Input: dimensioned drawing with shaded views. Units: mm. Origin: part minimum x, y, z. A direction names the side the tool comes from. Round coordinates to 2 decimals unless told otherwise and drop trailing zeros. Order: outer loops, then holes, each group sorted by start corner. A loop starts at its lowest first (then second) coordinate and runs counter-clockwise, first axis right, second up. Notation, with made-up numbers: M -37,73 L 10,73 A15 cw 10,91 Z; hole C 85.5,21.25 d4. An arc over 180 degrees is marked long. Answer as CSV lines item,"result". Start each with the question number.
Item 1: Line query: line 1 (Z direction, x = 113, y = 8.75); line 2 (X direction, y = 7.25, z = 78); line 3 (Y direction, x = 22, z = 23.5). Output: solid intervals per line, ascending. Write a range as [from, to].
Item 2: Set-up query: the marked faces 1 and 2. Return all of +Z, -Z, +X, -X, +Y, -Y with unobstructed straight access to the full face (end or side cutting, diameter ignored); none if empty.
Item 3: Section query D-D on z = 21.5. Return the cut outline in (x, y).
Item 4: Section query C-C on x = 7. Return the cut outline in (y, z).
Item 5: First-contact query: P1, Ø1, axis at x = 7.5, z = 77, coming from the +Y side; P2, Ø3, axis at x = 7, z = 7, coming from the -Y side. Flat tips, straight axial feed; report the tip coordinate or a pass-through.
Item 6: Section query B-B on z = 7. Return the cut outline in (x, y).
Item 7: Section query A-A on y = 5.75. Return the cut outline in (x, z), plus the area to 3 significant figures.
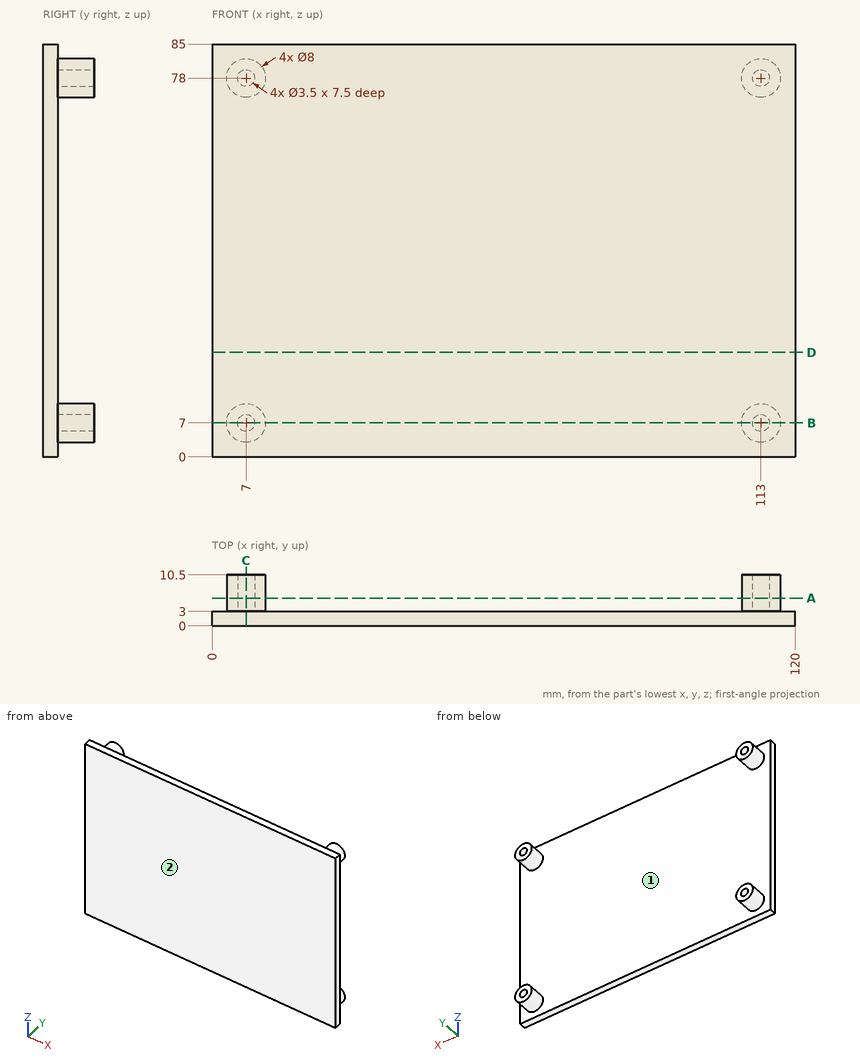
Results:
1,line 1,"[3, 5.25], [8.75, 11], [74, 76.25], [79.75, 82]"
1,line 2,"[3, 5.25], [8.75, 11], [109, 111.25], [114.75, 117]"
1,line 3,"[0, 3]"
2,face 1,"+Y"
2,face 2,"+Z, -Z, +X, -X, -Y"
3,outline,"M 0,0 L 120,0 L 120,3 L 0,3 Z"
4,outline,"M 0,0 L 3,0 L 3,3 L 10.5,3 L 10.5,5.25 L 3,5.25 L 3,8.75 L 10.5,8.75 L 10.5,11 L 3,11 L 3,74 L 10.5,74 L 10.5,76.25 L 3,76.25 L 3,79.75 L 10.5,79.75 L 10.5,82 L 3,82 L 3,85 L 0,85 Z"
5,P1,"y = 3"
5,P2,"y = 0"
6,outline,"M 0,0 L 120,0 L 120,3 L 117,3 L 117,10.5 L 114.75,10.5 L 114.75,3 L 111.25,3 L 111.25,10.5 L 109,10.5 L 109,3 L 11,3 L 11,10.5 L 8.75,10.5 L 8.75,3 L 5.25,3 L 5.25,10.5 L 3,10.5 L 3,3 L 0,3 Z"
7,outline,"C 7,7 d8; C 7,78 d8; C 113,7 d8; C 113,78 d8; hole C 7,7 d3.5; hole C 7,78 d3.5; hole C 113,7 d3.5; hole C 113,78 d3.5"
7,area,"163 mm^2"
